Part model, mm, in its own coordinate system. Face numbers are marked on the shaded views. A direction names the side the tool comes from. Coordinates: 2 decimals unless noted, no trailing zeros. Order: outer loops, then holes, each group sorted by start corner. A loop starts at its lowest first (then second) coordinate and runs counter-clockwise, first axis right, second up. Notation, with made-up numbers: M -28,89 L -3,89 A13 ccw -3,93 Z; hole C -3.75,-5.75 d11. An arc over 180 degrees is marked long. Answer in a Markdown table with one row per item. Add a question column.
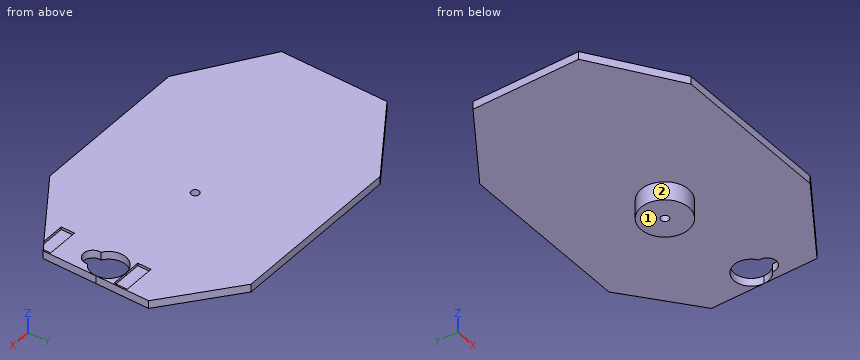
from build123d import *

# Parameters (mm, degrees)
BOX003_W          = 12
BOX003_H          = 5
BOX003_DEPTH      = 9
BOX002_W          = 12
BOX002_H          = 5
BOX002_DEPTH      = 9
CYLINDER007_R     = 3.5
CYLINDER007_DEPTH = 10
CYLINDER006_R     = 6.5
CYLINDER006_DEPTH = 10
BOX001_W          = 11
BOX001_H          = 4
BOX001_DEPTH      = 9
CYLINDER005_R     = 1.5
CYLINDER005_DEPTH = 20
PAD003_DEPTH      = 3
CYLINDER001_R     = 9
CYLINDER001_DEPTH = 9


with BuildPart() as cube003:
    # Box003 → Box003 (new body)
    with BuildSketch(Plane(origin=(37.5, -22.5, 9), x_dir=(1, 0, 0), z_dir=(0, 0, 1))):
        with Locations((6, 2.5)):
            Rectangle(BOX003_W, BOX003_H)
    extrude(amount=BOX003_DEPTH)


with BuildPart() as fusion006:
    # Box002 → Box002 (new body)
    with BuildSketch(Plane(origin=(37.5, 6.5, 9), x_dir=(1, 0, 0), z_dir=(0, 0, 1))):
        with Locations((6, 2.5)):
            Rectangle(BOX002_W, BOX002_H)
    extrude(amount=BOX002_DEPTH)

    # Fusion006: union Cube003
    add(cube003.part)


with BuildPart() as cylinder007:
    # Cylinder007 → Cylinder007 (new body)
    with BuildSketch(Plane(origin=(43.5, -6, 3), x_dir=(1, 0, 0), z_dir=(0, 0, 1))):
        Circle(CYLINDER007_R)
    extrude(amount=CYLINDER007_DEPTH)


with BuildPart() as fusion005:
    # Cylinder006 → Cylinder006 (new body)
    with BuildSketch(Plane(origin=(43.5, 0, 3), x_dir=(1, 0, 0), z_dir=(0, 0, 1))):
        Circle(CYLINDER006_R)
    extrude(amount=CYLINDER006_DEPTH)

    # Fusion005: union Cylinder007
    add(cylinder007.part)


with BuildPart() as cube001:
    # Box001 → Box001 (new body)
    with BuildSketch(Plane(origin=(38, 7, 9), x_dir=(1, 0, 0), z_dir=(0, 0, 1))):
        with Locations((5.5, 2)):
            Rectangle(BOX001_W, BOX001_H)
    extrude(amount=BOX001_DEPTH)


with BuildPart() as clone_of_cube001:
    # Clone001 base: copy of Cube001
    add(cube001.part)


with BuildPart() as clone_of_cube001_1:
    # Clone001 placement: moved
    add(clone_of_cube001.part.moved(Location((0, -29, 0))))


with BuildPart() as cylinder005:
    # Cylinder005 → Cylinder005 (new body)
    with BuildSketch(Plane.XY.offset(-4)):
        Circle(CYLINDER005_R)
    extrude(amount=CYLINDER005_DEPTH)


with BuildPart() as pad003:
    # Sketch003 → Pad003 (new body)
    with BuildSketch(Plane(origin=(-30, 0, 7), x_dir=(1, 0, 0), z_dir=(0, 0, 1))):
        Polygon((-40, 20), (-10, 40), (55, 40), (80, 20), (80, -20), (50, -40), (-10, -40), (-40, -20), align=None)
    extrude(amount=PAD003_DEPTH)


with BuildPart() as top_panel001:
    # Cylinder001 → Cylinder001 (new body)
    with BuildSketch(Plane.XY):
        Circle(CYLINDER001_R)
    extrude(amount=CYLINDER001_DEPTH)

    # Fusion003: union Pad003
    add(pad003.part)

    # Cut004: cut Cylinder005
    add(cylinder005.part, mode=Mode.SUBTRACT)

    # Fusion004: union Cube001, Clone of Cube001
    add(cube001.part)
    add(clone_of_cube001_1.part)

    # Cut005: cut Fusion005
    add(fusion005.part, mode=Mode.SUBTRACT)

    # Cut006: cut Fusion006
    add(fusion006.part, mode=Mode.SUBTRACT)


solid = top_panel001.part
(1) Slice it at B-B (y = 5). List the corners of the cut face in (x, z), and give its area (3 significant figures).
(2) 3-axis set-ups, long thin cutter, end or side, ignore diameter. For the marked faces 1 and 2: which of +Z, -Z, +X, -X, +Y, -Y reach the whole face in a straight line?
(3) Drop flat-ended pins along their axis: P1, Ø6, axis at x = 36, z = 3, coming from the -Y side; P2, Ø6, axis at y = -24, z = 5.5, coming from the +X side; P3, Ø6, axis at y = -8.5, z = 2, coming from the +X side; P4, Ø1.5, axis at x = 42, y = -20, coming from the +Z side. Give the stop position or say it passes through.
(4) Slice it at C-C (z = 5.5). List the corners of the cut face in (x, y), and give its area (3 significant figures).
(5) Slice it at A-A (x = 0). List the corners of the cut face in (y, z).
(6) Slice it at D-D (y = -35). List the corners of the cut face in (x, z).
(7) Wall check: line 1 (X direction, y = -6, z = 8.65); line 2 (X direction, y = 0, z = 5.25); line 3 (Y direction, x = 43.5, z = 7.65). Give the ranges that are in metal, low to high.
Computed:
| question | item | result |
|---|---|---|
| 1 | outline | M -70,7 L -7.48,7 L -7.48,0 L 7.48,0 L 7.48,7 L 39.35,7 L 39.35,10 L -70,10 Z; M 47.65,7 L 50,7 L 50,10 L 47.65,10 Z |
| 1 | area | 440 mm^2 |
| 2 | face 1 | -Z, +X, -X, +Y, -Y |
| 2 | face 2 | -Z |
| 3 | P1 | passes through |
| 3 | P2 | stops at x = 47.9 |
| 3 | P3 | stops at x = 7.12 |
| 3 | P4 | stops at z = 9 |
| 4 | outline | C 0,0 d18; hole C 0,0 d3 |
| 4 | area | 247 mm^2 |
| 5 | outline | M -40,7 L -9,7 L -9,0 L -1.5,0 L -1.5,10 L -40,10 Z; M 1.5,0 L 9,0 L 9,7 L 40,7 L 40,10 L 1.5,10 Z |
| 6 | outline | M -47.5,7 L 27.5,7 L 27.5,10 L -47.5,10 Z |
| 7 | line 1 | x = -70 to 40, 47 to 50 |
| 7 | line 2 | x = -9 to -1.5, 1.5 to 9 |
| 7 | line 3 | y = -24.33 to -9.5, 6.5 to 25.2 |
